Can you work these out from the model? Positions are in its coordinate system, mm. Face numbers are marked on the shaded views. A direction names the side the tool comes from. Round coordinates to 2 decimals unless told otherwise and drop trailing zeros. Loops run counter-clockwise (first coordinate to the right, second up) from the corner with the lowest first, then second, coordinate; pieces in that order, holes last. Notation, with made-up numbers: M -22,53 L -17,53 A12 cw -17,64 Z; hole C 29.5,56.5 d2. An arc over 180 degrees is marked long. Answer as CSV lines item,"result".
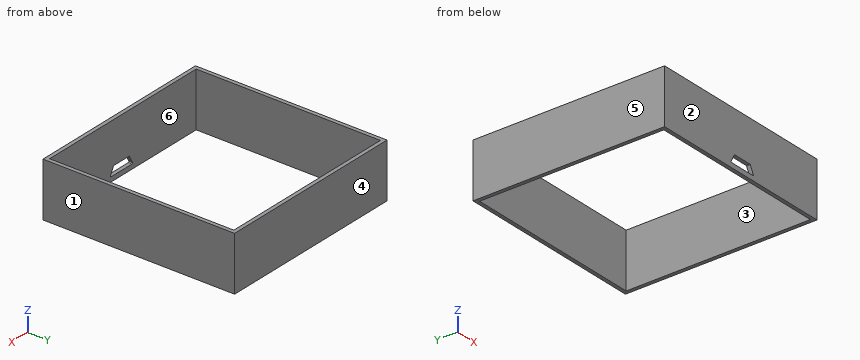
from build123d import *

# Parameters (mm, degrees)
F0_W     = 52
F0_H     = 52
F0_W_2   = 50
F0_H_2   = 50
F4_DEPTH = 14.8
F2_DEPTH = 1
F3_R     = 0.2


with BuildPart() as f4:
    # F0 (on Top) → F4 (new body)
    with BuildSketch(Plane.XY):
        with Locations((22.309654, -19.803896)):
            Rectangle(F0_W, F0_H)
        with Locations((22.309654, -19.803896)):
            Rectangle(F0_W_2, F0_H_2, mode=Mode.SUBTRACT)
    extrude(amount=F4_DEPTH)

    # F1 (on face) → F2 (cut, through all)
    with BuildSketch(Plane.XZ.offset(45.803896)):
        Polygon((18.909654, 1.248189), (22.309654, 1.248189), (26.709654, 1.248189), (25.509654, 3.598189), (22.809654, 3.598189), (20.109654, 3.598189), align=None)
    extrude(amount=-F2_DEPTH, mode=Mode.SUBTRACT)

    # F3
    f3_edges = [f4.edges().sort_by_distance(p)[0] for p in [
        (18.909654, -45.303896, 1.248189),
        (26.709654, -45.303896, 1.248189),
        (25.509654, -45.303896, 3.598189),
        (20.109654, -45.303896, 3.598189),
    ]]
    fillet(f3_edges, radius=F3_R)


solid = f4.part
Item 1: On a 3-axis mill with a long thin cutter (end or side, diameter ignored), from which of +Z, -Z, +X, -X, +Y, -Y can I reach the whole of each face in a straight line? I mean the marked faces 5 and 6. Say none if no direction works.
Output:
face 5,"+Z, -Z, -X, +Y, -Y"
face 6,"+Z, -Z"
Item 2: We'd pull the mould along Y, two halves only. Please class the marked faces 1, 2, 3 and 4: released by +Y, released by -Y, zero draft, split by the parting line, or undercut.
Output:
face 1,"zero draft"
face 2,"released by -Y"
face 3,"undercut"
face 4,"released by +Y"
Item 3: If we section it at B-B on x = 45: Write out the boundary of the cut face in (y, z).
Output:
outline,"M -45.8,0 L -44.8,0 L -44.8,14.8 L -45.8,14.8 Z; M 5.2,0 L 6.2,0 L 6.2,14.8 L 5.2,14.8 Z"
Item 4: If we section it at D-D on z = 2.75: Write out the boundary of the cut face in (x, y).
Output:
outline,"M -3.69,-45.8 L 19.68,-45.8 L 19.68,-44.8 L -2.69,-44.8 L -2.69,5.2 L 47.31,5.2 L 47.31,-44.8 L 25.94,-44.8 L 25.94,-45.8 L 48.31,-45.8 L 48.31,6.2 L -3.69,6.2 Z"
Item 5: If we section it at C-C on y = 2: Write out the boundary of the cut face in (x, z).
Output:
outline,"M -3.69,0 L -2.69,0 L -2.69,14.8 L -3.69,14.8 Z; M 47.31,0 L 48.31,0 L 48.31,14.8 L 47.31,14.8 Z"
Item 6: If I drill on line 1 along X through (y, z) = (-3, 1); line 2 along Y through (x, z) = (33.5, 0.5), over which ranges is the centre line in solid material (lowest first)? Write a range as from..to.
Output:
line 1,"x = -3.69..-2.69, 47.31..48.31"
line 2,"y = -45.8..-44.8, 5.2..6.2"
Item 7: If we section it at A-A on z = 13.25: Write out the boundary of the cut face in (x, y).
Output:
outline,"M -3.69,-45.8 L 48.31,-45.8 L 48.31,6.2 L -3.69,6.2 Z; hole M -2.69,-44.8 L 47.31,-44.8 L 47.31,5.2 L -2.69,5.2 Z"
